Part model, mm, in its own coordinate system. Coordinates: 2 decimals unless noted, no trailing zeros. Loops run counter-clockwise (first coordinate to the right, second up) from the corner with the lowest first, then second, coordinate; pieces in that order, holes last. Notation, with made-up numbers: M -25.5,62 L 17.5,62 A10 ccw 17.5,70 Z; hole C 16.5,-18.5 d1. An arc over 180 degrees is marked long. Answer as a JSON object with one key per item and string values. Group by question number.
1. Drop flat-ended pins along their axis: pin 1 Ø3.5 at (x, z) = (-8, 8) entering from -Y; pin 2 Ø6.5 at (x, z) = (11.31, 0) entering from +Y; pin 3 Ø1.5 at (x, y) = (15.5, 0.5) entering from -Z; pin 4 Ø5.5 at (x, z) = (-11.31, 0) entering from +Y. Give the stop position or say it passes through.
2. Saw through at C-C on z = 21. Write the cut outline in (x, y), then the cut area to 3 significant figures.
3. Drill centre lines: L1, parallel to Z at x = 28, y = 1.45; L2, parallel to Z at x = 0, y = 0.55; L3, parallel to X at y = 2.4, z = -20.5. Where is each one in solid material? Low to high.
4. Mould opens along X. For faces 1 (the face through (-9.303, 0.523, -0.447)), 2 (the face through (66, 1, 32)), 3 (the face through (38, 0, 1)) say: released by +X, released by -X, zero draft, split by the parting line, or undercut.
5. Saw through at B-B on y = 1.8. Count the separate pieces of the cut face and the enclosed holes in it, then the cut area to 3 significant figures.
6. Saw through at A-A on x = 28. Write the cut outline in (y, z), then the cut area to 3 significant figures.
Autodesk Inventor part; units mm, degrees
ref_plane "YZ Plane" through (0, 0, 0) normal (1, 0, 0) x (0, 1, 0)
ref_plane "XZ Plane" through (0, 0, 0) normal (0, 1, 0) x (-1, 0, 0)
ref_plane "XY Plane" through (0, 0, 0) normal (0, 0, 1) x (1, 0, 0)
sketch "Sketch1" plane through (0, 0, 0) normal (0, 1, 0) x (-1, 0, 0)
  arc A0 (0, -16) -> (0, 16) centre (0, 0) ccw
  circle A1 centre (8, -8) radius 2
  circle A2 centre (11.3137, 0) radius 2
  circle A3 centre (8, 8) radius 2
  circle A4 centre (0, 11.3137) radius 2
  circle A5 centre (-8, 8) radius 2
  circle A6 centre (-11.3137, 0) radius 2
  circle A7 centre (-8, -8) radius 2
  circle A8 centre (0, -11.3137) radius 2
  line L0 (0, 16) -> (-18, 38)
  line L1 (-18, 38) -> (-72, 38)
  line L2 (-72, 38) -> (-72, -38)
  line L3 (-72, -38) -> (-18, -38)
  line L4 (-18, -38) -> (0, -16)
  arc A9 (0, 16) -> (0, -16) centre (0, 0) ccw construction
  point P0 (-72, 0)
  dimension "d0" = 32
  dimension "d1" = 4
  dimension "d2" = 8
  dimension "d3" = 8
  dimension "d6" = 360
  dimension "d10" = 76
  dimension "d11" = 72
  dimension "d13" = 18
extrude "Extrusion1" add sketch "Sketch1" along normal blind 3
sketch "Sketch2" plane through (0, 3, 0) normal (0, 1, 0) x (1, 0, 0)
  circle A0 centre (28, -21) radius 7
  circle A1 centre (28, -21) radius 21 construction
  line L0 (0, 0) -> (72, 0) construction
  line L1 (72, -38) -> (72, 38) construction
  circle A2 centre (28, 21) radius 7
  circle A3 centre (28, 21) radius 21 construction
  circle A4 centre (64, -21) radius 2
  circle A5 centre (64, 21) radius 2
  dimension "d14" = 14
  dimension "d15" = 42
  dimension "d16" = 21
  dimension "d17" = 28
  dimension "d18" = 4
  dimension "d19" = 36
extrude "Extrusion2" cut sketch "Sketch2" against normal through all
sketch "Sketch3" plane through (0, 3, 0) normal (0, 1, 0) x (1, 0, 0)
  circle A0 centre (-11.3137, 0) radius 2
  circle A1 centre (-8, 8) radius 2
  circle A2 centre (0, 11.3137) radius 2
  circle A3 centre (8, 8) radius 2
  circle A4 centre (11.3137, 0) radius 2
  circle A5 centre (8, -8) radius 2
  circle A6 centre (0, -11.3137) radius 2
  circle A7 centre (-8, -8) radius 2
  point P0 (0, 0)
hole "Hole1" at (-8, 3, 8) at (-11.3137, 3, 0) at (-8, 3, -8) at (0, 3, -11.3137) at (8, 3, -8) at (11.3137, 3, 0) at (8, 3, 8) at (0, 3, 11.3137) direction (0, -1, 0) diameter 4.12 end through all countersink diameter 8 countersink angle 90
chamfer "Chamfer1" distance 12 angle 45 2 edges at (72, 1.5, 38) (72, 1.5, -38)
properties part number "ClawBase" material "Aluminum 6061"
Outcome:
{
 "1": {"pin 1": "passes through", "pin 2": "stops at y = 2.25", "pin 3": "stops at z = -35.86", "pin 4": "stops at y = 1.75"},
 "2": {"outline": "M 4.09,0 L 21,0 L 21,3 L 4.09,3 Z; M 35,0 L 62,0 L 62,3 L 35,3 Z; M 66,0 L 72,0 L 72,3 L 66,3 Z", "area": "150 mm²"},
 "3": {"L1": "z = -38 to -28, -14 to 14, 28 to 38", "L2": "z = -16 to -13.37, -9.25 to 9.25, 13.37 to 16", "L3": "x = 3.68 to 21.02, 34.98 to 62.06, 65.94 to 72"},
 "4": {"face 1": "undercut", "face 2": "released by +X", "face 3": "zero draft"},
 "5": {"separate pieces": "1", "enclosed holes": "12", "area": "4,800 mm²"},
 "6": {"outline": "M 0,-38 L 3,-38 L 3,-28 L 0,-28 Z; M 0,-14 L 3,-14 L 3,14 L 0,14 Z; M 0,28 L 3,28 L 3,38 L 0,38 Z", "area": "144 mm²"}
}
